Geometry check sheet. Reference: the model listing, model coordinates, mm. A direction names the side the tool comes from. Round coordinates to 2 decimals unless told otherwise and drop trailing zeros. Loops run counter-clockwise (first coordinate to the right, second up) from the corner with the lowest first, then second, coordinate; pieces in that order, holes last. Notation, with made-up numbers: (12, 86.5) - (48, 86.5) arc R30 ccw to (48, 120.5) - close; hole circle Ø11 at (2.5, -39.5). An arc over 180 degrees is marked (long way). Answer as CSV lines item,"result". Start each with the question number.
1) Access from +Z, -Z, +X, -X, +Y, -Y to the whole of each face (thin tool, end or side, straight path). Record for faces 1 (the flat face through (64, -7, 12.7)), 2 (the flat face through (19, -10, 12.7)), 3 (the cylindrical face through (37.836, -12.878, 42.505)).
2) Cross-section at A-A on y = -17.5. Record the boundary of the cut face in (x, z).
3) Cross-section at B-B on z = 17.5. Record the boundary of the cut face in (x, y), and give its area (3 significant figures).
4) Draft check along X on faces 4 (the cylindrical face through (67.691, -15.534, 6.439)), 5 (the flat face through (38, -13, 0)), 6 (the cylindrical face through (18.74, -15.22, 6.44)), 7 (the flat face through (50.8, -9.7, 15.6)). Enter one of: released by +X, released by -X, zero draft, split by the parting line, or undercut.
5) Depth check by flat-ended pin: P1, Ø11, axis at x = 62.07, y = -13.2, coming from the -Z side; P2, Ø3, axis at x = 34.5, y = -20.5, coming from the +Z side; P3, Ø1, axis at x = 11, y = -22.5, coming from the +Z side; P4, Ø8, axis at y = -20.5, z = 9.5, coming from the +X side. Enter the tip coordinate at first touch or a pass-through.
6) Cross-section at C-C on x = 64. Record the boundary of the cut face in (y, z), and give its area (3 significant figures).
7) Thickness scan on line 1 along Y through (x, z) = (44.5, 22); line 2 along X through (y, z) = (-15, 12); line 3 along Z through (x, y) = (8, -20.75). Record the ranges inside material, lowest first.
8) Cross-section at D-D on x = 27. Record the boundary of the cut face in (y, z).
from build123d import *

# Parameters (mm, degrees)
F1_DEPTH  = 25.4
F3_DEPTH  = 25.4
F5_DEPTH  = 25.4
F7_DEPTH  = 25.4
F8_R      = 6.567991
F9_DEPTH  = 25.4
F10_R     = 6.086179
F11_DEPTH = 25.4
F12_R     = 6.384731
F13_DEPTH = 25.4


with BuildPart() as f1:
    # F0 (on Front) → F1 (new body)
    with BuildSketch(Plane.XZ):
        Polygon((0, 12.7), (0, 0), (76.2, 0), (76.2, 12.7), (50.8, 12.7), (50.8, 44.45), (25.4, 44.45), (25.4, 12.7), align=None)
    extrude(amount=F1_DEPTH)

    # F2 (on face) → F3 (cut)
    with BuildSketch(Plane.XZ.offset(25.4)):
        with BuildLine():
            ThreePointArc((25.4, 30.930717), (38.1, 42.507362), (50.8, 30.930717))
            Line((50.8, 30.930717), (50.8, 44.45))
            Line((50.8, 44.45), (25.4, 44.45))
            Line((25.4, 44.45), (25.4, 30.930717))
        make_face()
    extrude(amount=-F3_DEPTH, mode=Mode.SUBTRACT)

    # F4 (on face) → F5 (cut)
    with BuildSketch(Plane.XY.offset(12.7)):
        with BuildLine():
            ThreePointArc((0, -10.345371), (3.606994, -3.535954), (10.453569, 0))
            Line((10.453569, 0), (0, 0))
            Line((0, 0), (0, -10.345371))
        make_face()
        with BuildLine():
            ThreePointArc((10.453569, -25.4), (3.606994, -21.864046), (0, -15.054629))
            Line((0, -15.054629), (0, -25.4))
            Line((0, -25.4), (10.453569, -25.4))
        make_face()
    extrude(amount=-F5_DEPTH, mode=Mode.SUBTRACT)

    # F6 (on face) → F7 (cut)
    with BuildSketch(Plane.XY.offset(12.7)):
        with BuildLine():
            ThreePointArc((66.74201, 0), (76.021911, -11.988349), (68.953343, -25.4))
            Line((68.953343, -25.4), (76.2, -25.4))
            Line((76.2, -25.4), (76.2, 0))
            Line((76.2, 0), (66.74201, 0))
        make_face()
    extrude(amount=-F7_DEPTH, mode=Mode.SUBTRACT)

    # F8 (on face) → F9 (cut)
    with BuildSketch(Plane.XY.offset(12.7)):
        with Locations((12.676189, -12.7)):
            Circle(F8_R)
    extrude(amount=-F9_DEPTH, mode=Mode.SUBTRACT)

    # F10 (on face) → F11 (cut)
    with BuildSketch(Plane.XY.offset(12.7)):
        with Locations((62.069037, -13.20309)):
            Circle(F10_R)
    extrude(amount=-F11_DEPTH, mode=Mode.SUBTRACT)

    # F12 (on face) → F13 (cut)
    with BuildSketch(Plane(origin=(25.4, 0, 0), x_dir=(0, -1, 0), z_dir=(-1, 0, 0))):
        with Locations((12.376302, 21.793298)):
            Circle(F12_R)
    extrude(amount=-F13_DEPTH, mode=Mode.SUBTRACT)


solid = f1.part
Answer block:
1,face 1,"+Z, +X, +Y, -Y"
1,face 2,"+Z, -X, +Y, -Y"
1,face 3,"+Z, +Y, -Y"
2,outline,"(0.71, 0) - (8.19, 0) - (8.19, 12.7) - (0.71, 12.7) - close; (17.16, 0) - (57.76, 0) - (57.76, 12.7) - (50.8, 12.7) - (50.8, 17.98) - (25.4, 17.98) - (25.4, 12.7) - (17.16, 12.7) - close; (25.4, 25.6) - (50.8, 25.6) - (50.8, 30.93) arc R12.75 ccw to (25.4, 30.93) - close; (66.38, 0) - (75.4, 0) - (75.4, 12.7) - (66.38, 12.7) - close"
3,outline,"(25.4, -25.4) - (50.8, -25.4) - (50.8, -17.1) - (25.4, -17.1) - close; (25.4, -7.65) - (50.8, -7.65) - (50.8, 0) - (25.4, 0) - close"
3,area,"405 mm^2"
4,face 4,"undercut"
4,face 5,"zero draft"
4,face 6,"undercut"
4,face 7,"released by +X"
5,P1,"passes through"
5,P2,"stops at z = 42.33"
5,P3,"stops at z = 12.7"
5,P4,"stops at x = 75.68"
6,outline,"(-25.4, 0) - (-18.97, 0) - (-18.97, 12.7) - (-25.4, 12.7) - close; (-7.43, 0) - (0, 0) - (0, 12.7) - (-7.43, 12.7) - close"
6,area,"176 mm^2"
7,line 1,"y = -25.4 to -18.76, -5.99 to 0"
7,line 2,"x = 0 to 6.52, 18.83 to 56.25, 67.88 to 75.96"
7,line 3,"z = 0 to 12.7"
8,outline,"(-25.4, 0) - (0, 0) - (0, 36.04) - (-25.4, 36.04) - close; hole circle Ø12.77 at (-12.38, 21.79)"
